For this review, take the finished solid that the model builds, in its own axes (mm). Face numbers are marked on the shaded views. A direction names the side the tool comes from. Give positions to 0.01 mm unless a question says otherwise; leave off trailing zeros. Order: outer loops, then holes, each group sorted by start corner. A loop starts at its lowest first (then second) coordinate and runs counter-clockwise, first axis right, second up.
from build123d import *

# Parameters (mm, degrees)
BOSS_EXTRUDE1_DEPTH  = 10
SKETCH2_W            = 32
SKETCH2_H            = 14
HOLE1_D              = 16.05
HOLE1_DEPTH          = 42
M5_CLEARANCE_HOLE1_D = 5.3
CIRPATTERN1_COUNT    = 3
CIRPATTERN1_ANGLE    = 90
MIRROR1_COPY_1_D     = 5.3
MIRROR1_COPY_2_D     = 5.3


with BuildPart() as part:
    # Sketch1 → Boss-Extrude1 (new body)
    with BuildSketch(Plane(origin=(0, 0, 0), x_dir=(0, -1, 0), z_dir=(-1, 0, 0))):
        with BuildLine():
            Line((20, -13.266499161), (20, 13.266499161))
            ThreePointArc((20, 13.266499161), (0, 24), (-20, 13.266499161))
            Line((-20, 13.266499161), (-20, -13.266499161))
            ThreePointArc((-20, -13.266499161), (0, -24), (20, -13.266499161))
        make_face()
    extrude(amount=-BOSS_EXTRUDE1_DEPTH)

    # Sketch2 → Revolve1 (revolve)
    with BuildSketch(Plane.XY):
        with Locations((26, 7)):
            Rectangle(SKETCH2_W, SKETCH2_H)
    revolve(axis=Axis((10, 0, 0), (1, 0, 0)))

    # Hole1
    with Locations(Plane(origin=(42, 0, 0), x_dir=(0, 0, -1), z_dir=(1, 0, 0))):
        with Locations((0, 0)):
            Hole(HOLE1_D / 2, depth=HOLE1_DEPTH)

    # M5 Clearance Hole1 (through all)
    with Locations(Plane(origin=(10, 0, 0), x_dir=(0, 0, -1), z_dir=(1, 0, 0))):
        with Locations((-13.435028843, -13.435028843)):
            m5_clearance_hole1 = Hole(M5_CLEARANCE_HOLE1_D / 2)

    # CirPattern1: M5 Clearance Hole1 ×3 about axis
    cirpattern1_axis = Axis((0, 0, 0), (-1, 0, 0))
    for i in range(1, CIRPATTERN1_COUNT):
        add(m5_clearance_hole1.rotate(cirpattern1_axis, i * CIRPATTERN1_ANGLE / (CIRPATTERN1_COUNT - 1)), mode=Mode.SUBTRACT)

    # Mirror1: M5 Clearance Hole1 across plane
    add(m5_clearance_hole1.mirror(Plane.XY), mode=Mode.SUBTRACT)

    # Mirror1 copy 1 (through all)
    with Locations(Plane(origin=(10, 0, 0), x_dir=(0, -0.707106781, 0.707106781), z_dir=(1, 0, 0))):
        with Locations((-13.435028843, 13.435028843)):
            Hole(MIRROR1_COPY_1_D / 2)

    # Mirror1 copy 2 (through all)
    with Locations(Plane(origin=(10, 0, 0), x_dir=(0, -1, 0), z_dir=(1, 0, 0))):
        with Locations((-13.435028843, 13.435028843)):
            Hole(MIRROR1_COPY_2_D / 2)


solid = part.part
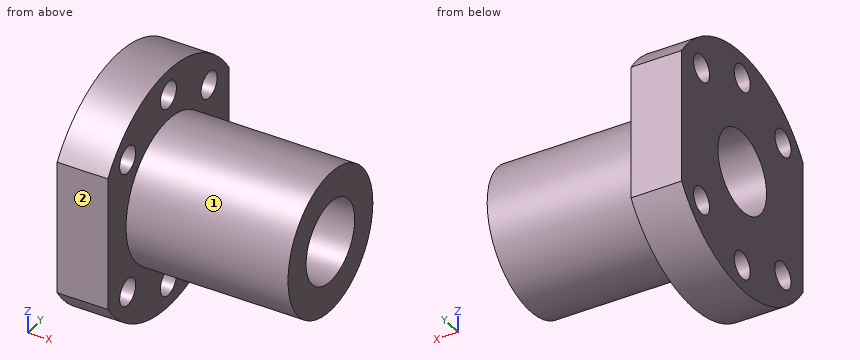
1) We need section C-C on x = 36.5. Give the boundary of the cut face in (y, z) (3 decimals).
Answer sheet:
outline: circle Ø28 at (0, 0); hole circle Ø16.05 at (0, 0)
2) To check wall thickness, follow line 1 (X direction, y = -11, z = 10); line 2 (Z direction, x = 11, y = 4.5); line 3 (Y direction, x = 4, z = -19). State the ranges of each line that lie inside material, in increasing order.
Answer sheet:
line 1: x = 0 to 10
line 2: z = -13.26 to -6.64, 6.64 to 13.26
line 3: y = -14.66 to -2.65, 2.65 to 14.66
3) We need section A-A on z = 0. Give the boundary of the cut face in (x, y) (3 decimals).
Answer sheet:
outline: (0, -20) - (10, -20) - (10, -14) - (42, -14) - (42, -8.025) - (0, -8.025) - close; (0, 8.025) - (42, 8.025) - (42, 14) - (10, 14) - (10, 20) - (0, 20) - close
4) Tool access review of the marked faces 1 and 2: name each direction out of +Z, -Z, +X, -X, +Y, -Y from which nothing blocks a thin tool from reaching the whole face with its end or side.
Answer sheet:
face 1: +X
face 2: +Z, -Z, +X, -X, -Y
5) We need section B-B on y = -3.5. Give the boundary of the cut face in (x, z), then the cut area to 3 significant figures.
Answer sheet:
outline: (0, -23.74) - (10, -23.74) - (10, -13.56) - (42, -13.56) - (42, -7.22) - (0, -7.22) - close; (0, 7.22) - (42, 7.22) - (42, 13.56) - (10, 13.56) - (10, 23.74) - (0, 23.74) - close
area: 736 mm2
6) We need section D-D on z = 11.5. Give the boundary of the cut face in (x, y), then the cut area to 3 significant figures.
Answer sheet:
outline: (0, -20) - (10, -20) - (10, -15.25) - (0, -15.25) - close; (0, -11.62) - (10, -11.62) - (10, -7.98) - (42, -7.98) - (42, 7.98) - (10, 7.98) - (10, 11.62) - (0, 11.62) - close; (0, 15.25) - (10, 15.25) - (10, 20) - (0, 20) - close
area: 839 mm2
7) Clearance check with flat-ended pins moving along their axes: pin 1 (7 mm diameter, centred on y = -13.44, z = -13.44, fed in from +X); pin 2 (12 mm diameter, centred on x = 14, z = -1.5, fed in from -Y); pin 3 (6 mm diameter, centred on x = 18.5, y = 7, fed in from -Z); pin 4 (8 mm diameter, centred on x = 26, z = 15, fed in from -Y). State where each tip first meets the part, or that it passes through.
Answer sheet:
pin 1: stops at x = 10
pin 2: stops at y = -20
pin 3: stops at z = -13.42
pin 4: stops at y = -8.66
